Autodesk Inventor part; units mm, degrees
ref_plane "YZ Plane" through (0, 0, 0) normal (1, 0, 0) x (0, 1, 0)
ref_plane "XZ Plane" through (0, 0, 0) normal (0, 1, 0) x (-1, 0, 0)
ref_plane "XY Plane" through (0, 0, 0) normal (0, 0, 1) x (1, 0, 0)
sketch "Sketch1" plane through (0, 0, 0) normal (0, 1, 0) x (-1, 0, 0)
  circle A0 centre (24.1, 110.65) radius 0.25
  circle A1 centre (-70.5, 110.65) radius 0.25
  circle A2 centre (-45.6, 89.15) radius 0.25
  circle A3 centre (0, 67.65) radius 0.25
  circle A4 centre (70.5, 42.15) radius 0.25
  circle A5 centre (32.15, 17.15) radius 0.25
  circle A6 centre (60.5, -17.65) radius 0.25
  circle A7 centre (-60.5, -17.65) radius 0.25
  circle A8 centre (24.1, -67.65) radius 0.25
  circle A9 centre (-70.5, -67.65) radius 0.25
  circle A10 centre (-45.6, -89.15) radius 0.25
  circle A11 centre (0, -110.65) radius 0.25
  circle A12 centre (-70.5, -110.65) radius 0.25
  circle A13 centre (70.5, -110.65) radius 0.25
  circle A14 centre (45.6, -89.15) radius 0.25
  circle A15 centre (-24.1, -67.65) radius 0.25
  circle A16 centre (70.5, -67.65) radius 0.25
  circle A17 centre (0, -17.65) radius 0.25
  circle A18 centre (-32.15, 17.15) radius 0.25
  circle A19 centre (-70.5, 42.15) radius 0.25
  circle A20 centre (-70.5, 67.65) radius 0.25
  circle A21 centre (70.5, 67.65) radius 0.25
  circle A22 centre (45.6, 89.15) radius 0.25
  circle A23 centre (-24.1, 110.65) radius 0.25
  circle A24 centre (70.5, 110.65) radius 0.25
  line L0 (75.5, -115.65) -> (75.5, -62.65)
  line L1 (75.5, -62.65) -> (65.5, -42.65)
  line L2 (65.5, -42.65) -> (65.5, 22.15)
  line L3 (65.5, 22.15) -> (75.5, 42.15)
  line L4 (75.5, 42.15) -> (75.5, 115.65)
  line L5 (75.5, 115.65) -> (30.5, 135.65)
  line L6 (30.5, 135.65) -> (-30.5, 135.65)
  line L7 (-30.5, 135.65) -> (-75.5, 115.65)
  line L8 (-75.5, 115.65) -> (-75.5, 42.15)
  line L9 (-75.5, 42.15) -> (-65.5, 22.15)
  line L10 (-65.5, 22.15) -> (-65.5, -42.65)
  line L11 (-65.5, -42.65) -> (-75.5, -62.65)
  line L12 (-75.5, -62.65) -> (-75.5, -115.65)
  line L13 (-75.5, -115.65) -> (-30.5, -135.65)
  line L14 (-30.5, -135.65) -> (30.5, -135.65)
  line L15 (30.5, -135.65) -> (75.5, -115.65)
  circle A25 centre (0, -110.65) radius 2
  circle A26 centre (70.5, -110.65) radius 2
  circle A27 centre (-70.5, -110.65) radius 2
  circle A28 centre (45.6, -89.15) radius 2
  circle A29 centre (-45.6, -89.15) radius 2
  circle A30 centre (70.5, -67.65) radius 2
  circle A31 centre (24.1, -67.65) radius 2
  circle A32 centre (-24.1, -67.65) radius 2
  circle A33 centre (-70.5, -67.65) radius 2
  circle A34 centre (60.5, -17.65) radius 2
  circle A35 centre (0, -17.65) radius 2
  circle A36 centre (-32.15, 17.15) radius 2
  circle A37 centre (-60.5, -17.65) radius 2
  circle A38 centre (32.15, 17.15) radius 2
  circle A39 centre (70.5, 42.15) radius 2
  circle A40 centre (-70.5, 42.15) radius 2
  circle A41 centre (-70.5, 67.65) radius 2
  circle A42 centre (0, 67.65) radius 2
  circle A43 centre (70.5, 67.65) radius 2
  circle A44 centre (45.6, 89.15) radius 2
  circle A45 centre (-45.6, 89.15) radius 2
  circle A46 centre (-70.5, 110.65) radius 2
  circle A47 centre (-24.1, 110.65) radius 2
  circle A48 centre (24.1, 110.65) radius 2
  circle A49 centre (70.5, 110.65) radius 2
  line L16 (30.5, 135.65) -> (-30.15, 135.65)
  circle A50 centre (30.5, 125.65) radius 1.5
  circle A51 centre (-30.15, 125.65) radius 1.5
  line L17 (30.5, -135.65) -> (-30.15, -135.65)
  circle A52 centre (30.5, -125.65) radius 1.5
  circle A53 centre (-30.15, -125.65) radius 1.5
  point P0 (0, 0)
  point P1 (0, 0)
  dimension "d0" = 4
  dimension "d1" = 4
  dimension "d2" = 4
  dimension "d3" = 4
  dimension "d4" = 4
  dimension "d5" = 4
  dimension "d6" = 4
  dimension "d7" = 4
  dimension "d8" = 4
  dimension "d9" = 4
  dimension "d10" = 4
  dimension "d11" = 4
  dimension "d12" = 4
  dimension "d13" = 4
  dimension "d14" = 4
  dimension "d15" = 4
  dimension "d16" = 4
  dimension "d17" = 4
  dimension "d18" = 4
  dimension "d19" = 4
  dimension "d20" = 4
  dimension "d21" = 4
  dimension "d22" = 4
  dimension "d23" = 4
  dimension "d24" = 4
  dimension "d28" = 3
  dimension "d29" = 3
  dimension "d31" = 3
  dimension "d32" = 3
extrude "Extrusion1" add sketch "Sketch1" along normal blind 2 contours L15 L14 L13 L12 L11 L10 L9 L8 L7 L6 L5 L4 L3 L2 L1 L0 | A50 | A51 | A52 | A53
extrude "Extrusion2" cut sketch "Sketch1" along normal blind 2 contours A50 | A51 | A52 | A53
properties part number "podvozek"
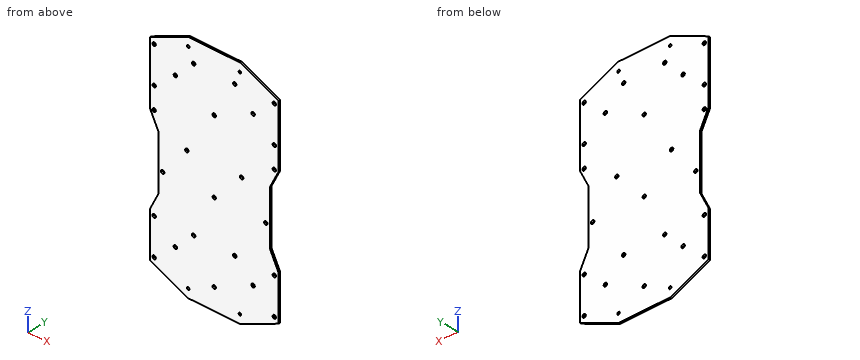
Work out the finished part from the listing and answer in its coordinate system (mm). Round coordinates to 2 decimals unless told otherwise and drop trailing zeros. Write each loop counter-clockwise with the first axis right and the second up, starting at its lowest first coordinate (ties: lowest second). Pieces come first, ordered by that corner, then holes. Notation, with made-up numbers: (63.25, -27.75) -> (105.25, -27.75) arc R16 ccw to (105.25, -23.75) -> close; hole circle Ø9 at (72.5, 29). An arc over 180 degrees is marked (long way). Answer as CSV lines item,"result". Start each with the question number.
(1) The part is cut by section B-B, the plane y = 1.3. Give the number of separate pieces and of enclosed holes in the cut face, then the cut area to 3 significant figures.
(2) Each of these flat-tipped pins is pushed along its axis until it touches: pin 1 (6.5 mm diameter, centred on x = 60.5, z = -17.65, fed in from +Y); pin 2 (1 mm diameter, centred on y = 0.5, z = -26.5, fed in from +X). Where does it stop, or does it pass through?
(3) The part is cut by section A-A, the plane z = -27.5. Give the vertices of the cut face in (x, y), then the cut area to 3 significant figures.
(4) Find the intervals of material crossed by probe 1 along Z at (x, y) = (-24.1, 0.8); probe 2 along Z at (x, y) = (23, 1.8); probe 3 along Z at (x, y) = (-30.5, 1.4), in increasing order.
(5) The part is cut by section C-C, the plane z = 31.5. Give the vertices of the cut face in (x, y) (3 decimals).
Output values:
1,separate pieces,"1"
1,enclosed holes,"29"
1,area,"37,100 mm²"
2,pin 1,"stops at y = 2"
2,pin 2,"stops at x = 65.5"
3,outline,"(-65.5, 0) -> (65.5, 0) -> (65.5, 2) -> (-65.5, 2) -> close"
3,area,"262 mm²"
4,probe 1,"z = -135.65 to -69.65, -65.65 to 108.65, 112.65 to 135.65"
4,probe 2,"z = -135.65 to -69.32, -65.98 to 108.98, 112.32 to 135.65"
4,probe 3,"z = -135.65 to -127.15, -124.15 to 16.02, 18.28 to 124.15, 127.15 to 135.65"
5,outline,"(-70.175, 0) -> (70.175, 0) -> (70.175, 2) -> (-70.175, 2) -> close"
